Can you work these out from the model? Positions are in its coordinate system, mm. Face numbers are marked on the shaded views. A direction names the side the tool comes from. Give positions to 0.01 mm unless a question says otherwise; leave off trailing zeros. Loops run counter-clockwise (first coordinate to the right, second up) from the corner with the lowest first, then second, coordinate; pieces in that order, holes last. Notation, with made-up numbers: (1.5, 54.5) - (57.5, 54.5) arc R5 ccw to (57.5, 63.5) - close; hole circle Ø7 at (60, -19.75). An arc over 180 degrees is marked (long way). Answer as a JSON object with one key per item and string values. Group by question number.
Item 1: Which directions (+Z, -Z, +X, -X, +Y, -Y) give clear straight access to the entire face, cutting with the end or side of a thin tool? Please do the marked faces 1 and 2.
Item 2: Suppose I cut it at A-A on x = 0. Write out the boundary of the cut face in (y, z).
Item 3: Please list where these lines run through material, in increasing order: L1, parallel to Z at x = 0, y = -5.5; L2, parallel to Y at x = -3.75, z = 10.75; L3, parallel to Y at x = 3.5, z = 12.
Item 4: Will these pins go through, and if not, where does the flat tip stop? pin 1 (8 mm diameter, centred on x = -8, z = 4.5, fed in from +Y); pin 2 (7 mm diameter, centred on x = 0, y = 0, fed in from +Z); pin 3 (1.5 mm diameter, centred on x = 2, z = 13, fed in from -Y).
Item 5: Thinking about a two-plate mould opening in X: for the marked faces 3, 4 and 5, which applies, pulls with the +X half, pulls with the -X half, needs draft (parallel to the pull), parting line crosses it, or undercut?
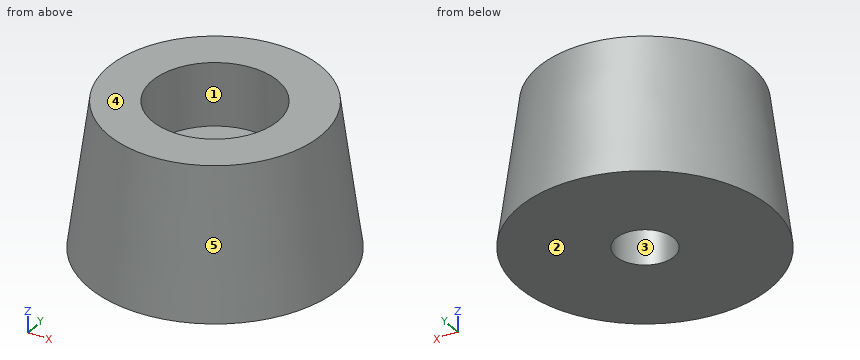
from build123d import *

# Parameters (mm, degrees)
SKETCH001_R     = 11
SKETCH_R        = 13
SKETCH002_R     = 3
POCKET_DEPTH    = 15.001
SKETCH003_R     = 6.5
POCKET001_DEPTH = 6.501


with BuildPart() as part:
    # Sketch001 (on DatumPlane) → AdditiveLoft section 0
    with BuildSketch(Plane.XY.offset(15)):
        Circle(SKETCH001_R)
    # Sketch → AdditiveLoft section 1
    with BuildSketch(Plane.XY):
        Circle(SKETCH_R)
    loft()

    # Sketch002 → Pocket (cut, through all)
    with BuildSketch(Plane.XY):
        Circle(SKETCH002_R)
    extrude(amount=POCKET_DEPTH, mode=Mode.SUBTRACT)

    # Sketch003 (on DatumPlane) → Pocket001 (cut, through all)
    with BuildSketch(Plane.XY.offset(8.5)):
        Circle(SKETCH003_R)
    extrude(amount=POCKET001_DEPTH, mode=Mode.SUBTRACT)


solid = part.part
Worked out:
{
 "1": {"face 1": "+Z", "face 2": "-Z, +X, -X, +Y, -Y"},
 "2": {"outline": "(-13, 0) - (-3, 0) - (-3, 8.5) - (-6.5, 8.5) - (-6.5, 15) - (-11, 15) - close; (3, 0) - (13, 0) - (11, 15) - (6.5, 15) - (6.5, 8.5) - (3, 8.5) - close"},
 "3": {"L1": "z = 0 to 8.5", "L2": "y = -10.94 to -5.31, 5.31 to 10.94", "L3": "y = -10.85 to -5.48, 5.48 to 10.85"},
 "4": {"pin 1": "stops at y = 11.85", "pin 2": "stops at z = 8.5", "pin 3": "stops at y = -11.24"},
 "5": {"face 3": "undercut", "face 4": "needs draft", "face 5": "parting line crosses it"}
}
